Check sheet for the modelled part. Datum: model origin and axes. Units: mm. A direction names the side the tool comes from. Give positions to 0.01 mm unless a question says otherwise; leave off trailing zeros. Order: outer loops, then holes, each group sorted by start corner. A loop starts at its lowest first (then second) coordinate and runs counter-clockwise, first axis right, second up.
```python
from build123d import *

# Parameters (mm, degrees)
SKETCH1_W           = 61
SKETCH1_H           = 30
BOSS_EXTRUDE1_DEPTH = 29
SKETCH2_W           = 7
SKETCH2_H           = 15
BOSS_EXTRUDE2_DEPTH = 17.5
FILLET1_R           = 2
FILLET2_R           = 2


with BuildPart() as part:
    # Sketch1 → Boss-Extrude1 (new body)
    with BuildSketch(Plane(origin=(0, 0, 0), x_dir=(1, 0, 0), z_dir=(0, 1, 0))):
        Rectangle(SKETCH1_W, SKETCH1_H)
    extrude(amount=BOSS_EXTRUDE1_DEPTH)

    # Sketch2 → Boss-Extrude2 (add)
    with BuildSketch(Plane.ZY.offset(30.5)):
        with Locations((-11.5, 14.5)):
            Rectangle(SKETCH2_W, SKETCH2_H)
    extrude(amount=BOSS_EXTRUDE2_DEPTH)

    # Fillet1
    fillet1_edges = [part.edges().sort_by_distance(p)[0] for p in [
        (-39.25, 22, -15),
        (-39.25, 7, -15),
        (-39.25, 7, -8),
        (-39.25, 22, -8),
    ]]
    fillet(fillet1_edges, radius=FILLET1_R)

    # Fillet2
    fillet2_edges = [part.edges().sort_by_distance(p)[0] for p in [
        (30.5, 14.5, -15),
        (0, 29, -15),
        (30.5, 29, 0),
        (-30.5, 29, 0),
        (30.5, 0, 0),
        (0, 0, -15),
        (-30.5, 0, 0),
        (-30.5, 14.5, 15),
        (0, 29, 15),
        (30.5, 14.5, 15),
        (0, 0, 15),
        (-30.5, 25.5, -15),
        (-30.5, 3.5, -15),
    ]]
    fillet(fillet2_edges, radius=FILLET2_R)


solid = part.part
```
(1) Sectioned sample at B-B (z = 5.25). Enter the section's corners in (x, y).
(2) Release check for a two-part mould opening along X. For faces 6 (the face through (29.93, 0.6, -0.18)), 7 (the face through (-48, 15, -12)), 8 (the face through (0, 0, 0)) record: released by +X, released by -X, zero draft, split by the parting line, or undercut.
(3) Sectioned sample at D-D (z = -10.75). Enter the section's corners in (x, y).
(4) Sectioned sample at C-C (x = -43). Enter the section's corners in (y, z), plus the area to 3 significant figures.
(5) Tool access check on faces 1 (the face through (-39.37, 7.57, -8.6)), 2 (the face through (-38.39, 7.6, -14.43)), 3 (the face through (-39, 14, -8)), 4 (the face through (-39.37, 21.4, -8.57)), 5 (the face through (-38.39, 21.4, -14.43)). Record the directions out of +Z, -Z, +X, -X, +Y, -Y that give a thin tool (end or side, any length) a straight path to the whole face; none if there is none.
(6) Thickness scan on L1, parallel to X at y = 20.25, z = 9; L2, parallel to X at y = 27.5, z = 10. Record the ranges inside material, lowest first.
(7) Go/stop test with flat-tipped pins: P1, Ø1, axis at y = 8, z = 9.5, coming from the -X side; P2, Ø2.5, axis at x = -37.5, z = -11.5, coming from the -Y side; P3, Ø12, axis at x = -41, y = 16, coming from the +Z side. Record where each tip stops, or that it passes through.
(8) Sectioned sample at A-A (y = 14.5). Enter the section's corners in (x, z).
Values follow:
1. outline: (-30.5, 2) arc R2 ccw to (-28.5, 0) - (28.5, 0) arc R2 ccw to (30.5, 2) - (30.5, 27) arc R2 ccw to (28.5, 29) - (-28.5, 29) arc R2 ccw to (-30.5, 27) - close
2. face 6: released by +X
2. face 7: released by -X
2. face 8: zero draft
3. outline: (-48, 7) - (-30.5, 7) - (-30.5, 2) arc R2 ccw to (-28.5, 0) - (28.5, 0) arc R2 ccw to (30.5, 2) - (30.5, 27) arc R2 ccw to (28.5, 29) - (-28.5, 29) arc R2 ccw to (-30.5, 27) - (-30.5, 22) - (-48, 22) - close
4. outline: (7, -13) arc R2 ccw to (9, -15) - (20, -15) arc R2 ccw to (22, -13) - (22, -10) arc R2 ccw to (20, -8) - (9, -8) arc R2 ccw to (7, -10) - close
4. area: 102 mm2
5. face 1: +Z, -X, -Y
5. face 2: -Z, -X, -Y
5. face 3: +Z, -X, +Y, -Y
5. face 4: +Z, -X, +Y
5. face 5: -Z, -X, +Y
6. L1: x = -30.5 to 30.5
6. L2: x = -30.44 to 30.44
7. P1: stops at x = -30.5
7. P2: stops at y = 7
7. P3: stops at z = -8
8. outline: (-48, -15) - (28.5, -15) arc R2 ccw to (30.5, -13) - (30.5, 13) arc R2 ccw to (28.5, 15) - (-28.5, 15) arc R2 ccw to (-30.5, 13) - (-30.5, -8) - (-48, -8) - close
